```python
from build123d import *

# Parameters (mm, degrees)
F0_W     = 101.6
F0_H     = 76.2
F1_DEPTH = 25.4
F3_DEPTH = 25.4
F4_DEPTH = 25.4


with BuildPart() as f1:
    # F0 (on Top) → F1 (new body)
    with BuildSketch(Plane.XY):
        with Locations((3.972126, -13.183172)):
            Rectangle(F0_W, F0_H)
    extrude(amount=-F1_DEPTH)

    # F2 (on face) → F3 (join)
    with BuildSketch(Plane.XY):
        Polygon((-46.827874, -51.283172), (-34.127874, -51.283172), (16.672126, 24.916828), (-46.827874, 24.916828), align=None)
    extrude(amount=F3_DEPTH)

    # F2 (on face) → F4 (join)
    with BuildSketch(Plane.XY):
        Polygon((54.772126, -13.183172), (35.323564, -51.283172), (54.772126, -51.283172), align=None)
    extrude(amount=F4_DEPTH)


solid = f1.part
```
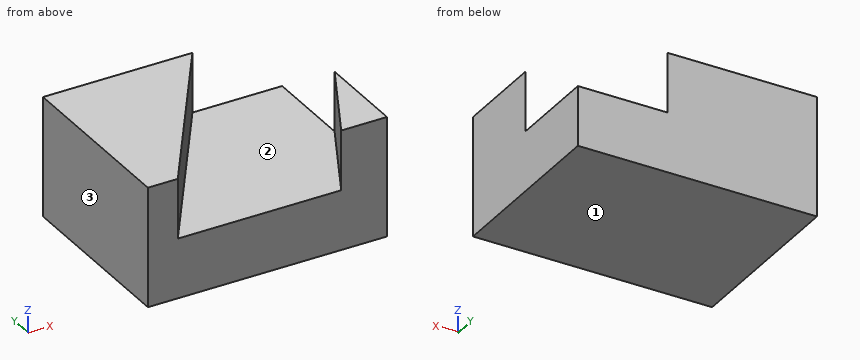
Can you work these out from the model? Positions are in its coordinate system, mm. Face numbers are marked on the shaded views. Give positions to 0.01 mm unless a question says otherwise; leave off trailing zeros. Loops run counter-clockwise (first coordinate to the right, second up) from the corner with the lowest first, then second, coordinate; pieces in that order, holes last. Notation, with made-up numbers: M 44,-27.75 L 94,-27.75 A16 ccw 94,-7.75 Z; hole C 10.5,-22 d9. An arc over 180 degrees is marked long. Use one line per item in the form item = value. Start each with the question number.
(1) I want a section at B-B, the plane y = -28. Write out the boundary of the cut face in (x, z).
(2) I want a section at D-D, the plane y = 18.5. Write out the boundary of the cut face in (x, z).
(3) I'm going to push a flat-ended pin straight in: P1, Ø1.5, axis at x = 27.5, y = -34.5, coming from the +Z side. Where does the tip first touch, or does it pass through?
(4) I want a section at A-A, the plane z = 16.5. Write out the boundary of the cut face in (x, y).
(5) Please list where these lines run through material, in increasing order: line 1 (X direction, y = -38.5, z = 23.5); line 2 (Z direction, x = 26.5, y = -16); line 3 (X direction, y = -29, z = 21.5).
(6) Thinking about a two-plate mould opening in X: for the marked faces 1, 2 and 3, which applies, released by +X, released by -X, zero draft, split by the parting line, or undercut?
(7) I want a section at C-C, the plane x = 5.5. Write out the boundary of the cut face in (y, z), and give its area (3 significant figures).
Worked out:
q1.outline = M -46.83,-25.4 L 54.77,-25.4 L 54.77,25.4 L 47.21,25.4 L 47.21,0 L -18.61,0 L -18.61,25.4 L -46.83,25.4 Z
q2.outline = M -46.83,-25.4 L 54.77,-25.4 L 54.77,0 L 12.39,0 L 12.39,25.4 L -46.83,25.4 Z
q3.P1 = 0
q4.outline = M -46.83,-51.28 L -34.13,-51.28 L 16.67,24.92 L -46.83,24.92 Z; M 35.32,-51.28 L 54.77,-51.28 L 54.77,-13.18 Z
q5.line_1 = -46.83 to -25.61, 41.85 to 54.77
q5.line_2 = -25.4 to 0
q5.line_3 = -46.83 to -19.27, 46.7 to 54.77
q6.face_1 = zero draft
q6.face_2 = undercut
q6.face_3 = released by -X
q7.outline = M -51.28,-25.4 L 24.92,-25.4 L 24.92,25.4 L 8.16,25.4 L 8.16,0 L -51.28,0 Z
q7.area = 2,360 mm²
